CAD build for the part. Positions are in the model's coordinates, mm. A direction names the side the tool comes from. Give positions to 0.01 mm unless a question says otherwise; leave off trailing zeros. Write each loop counter-clockwise with the first axis right and the second up, starting at its lowest first coordinate (ties: lowest second). Pieces come first, ordered by that corner, then holes. Notation, with made-up numbers: (-18.75, 89) - (37.25, 89) arc R19 cw to (37.25, 107) - close; hole circle Ø5 at (34.5, 28). An arc over 180 degrees is marked (long way). Answer as a JSON object with one key per item and string values.
from build123d import *

# Parameters (mm, degrees)
F2_R     = 25.25
F3_DEPTH = 2
F5_DEPTH = 2
F6_R     = 4.99999
F7_R     = 3


# Not quite as in the source:
# - a fillet or chamfer is up to 0.001 mm smaller than in the source, because OpenCascade refuses the exact size
# - a feature names something its author has since deleted; it is built from what else it names


with BuildPart() as f1:
    # F0 (on Top) → F1 (revolve)
    with BuildSketch(Plane.XY):
        Polygon((-18, 18.5), (-18, 13.5), (0, 13.5), (11.6913429511, 20.25), (25.1913429511, 20.25), (25.1913429511, 25.25), (10.3515969889, 25.25), (-1.3397459622, 18.5), align=None)
    revolve(axis=Axis((-8.7595172226, 0, 0), (1, 0, 0)))

    # F2 (on face) → F3 (join)
    with BuildSketch(Plane.YZ.offset(25.1913429511)):
        Circle(F2_R)
    extrude(amount=F3_DEPTH)

    # F4 (on face) → F5 (cut, through all)
    with BuildSketch(Plane.YZ.offset(27.1913429511)):
        with BuildLine():
            ThreePointArc((17, 11.0028405423), (15.1695473581, 13.4144449363), (13, 15.5261875552))
            Line((13, 15.5261875552), (13, -15.5261875552))
            ThreePointArc((13, -15.5261875552), (15.1695473581, -13.4144449363), (17, -11.0028405423))
            Line((17, -11.0028405423), (17, 11.0028405423))
        make_face()
        with BuildLine():
            ThreePointArc((12, 16.3114223782), (10.0654136275, 17.5712819255), (8, 18.6027551723))
            Line((8, 18.6027551723), (8, -18.6027551723))
            ThreePointArc((8, -18.6027551723), (10.0654136275, -17.5712819255), (12, -16.3114223782))
            Line((12, -16.3114223782), (12, 16.3114223782))
        make_face()
        with BuildLine():
            ThreePointArc((7, 19.0016446657), (5.0261919098, 19.6163170571), (3, 20.0265448842))
            Line((3, 20.0265448842), (3, -20.0265448842))
            ThreePointArc((3, -20.0265448842), (5.0261919098, -19.6163170571), (7, -19.0016446657))
            Line((7, -19.0016446657), (7, 19.0016446657))
        make_face()
        with BuildLine():
            ThreePointArc((2, 20.1509925314), (0, 20.25), (-2, 20.1509925314))
            Line((-2, 20.1509925314), (-2, -20.1509925314))
            ThreePointArc((-2, -20.1509925314), (0, -20.25), (2, -20.1509925314))
            Line((2, -20.1509925314), (2, 20.1509925314))
        make_face()
        with BuildLine():
            Line((-3, -20.0265448842), (-3, 20.0265448842))
            ThreePointArc((-3, 20.0265448842), (-5.0261919098, 19.6163170571), (-7, 19.0016446657))
            Line((-7, 19.0016446657), (-7, -19.0016446657))
            ThreePointArc((-7, -19.0016446657), (-5.0261919098, -19.6163170571), (-3, -20.0265448842))
        make_face()
        with BuildLine():
            Line((-8, -18.6027551723), (-8, 18.6027551723))
            ThreePointArc((-8, 18.6027551723), (-10.0654136275, 17.5712819255), (-12, 16.3114223782))
            Line((-12, 16.3114223782), (-12, -16.3114223782))
            ThreePointArc((-12, -16.3114223782), (-10.0654136275, -17.5712819255), (-8, -18.6027551723))
        make_face()
        with BuildLine():
            Line((-13, -15.5261875552), (-13, 15.5261875552))
            ThreePointArc((-13, 15.5261875552), (-15.1695473581, 13.4144449363), (-17, 11.0028405423))
            Line((-17, 11.0028405423), (-17, -11.0028405423))
            ThreePointArc((-17, -11.0028405423), (-15.1695473581, -13.4144449363), (-13, -15.5261875552))
        make_face()
        with BuildLine():
            Line((-18, -9.2769876576), (-18, 9.2769876576))
            ThreePointArc((-18, 9.2769876576), (-20.25, 0), (-18, -9.2769876576))
        make_face()
        with BuildLine():
            ThreePointArc((20.25, 0), (19.6794626451, 4.772970773), (18, 9.2769876576))
            Line((18, 9.2769876576), (18, -9.2769876576))
            ThreePointArc((18, -9.2769876576), (19.6794626451, -4.772970773), (20.25, 0))
        make_face()
    extrude(amount=-F5_DEPTH, mode=Mode.SUBTRACT)

    # F6 (radius 5 in the source; OpenCascade refuses exactly that, so slightly less here)
    f6_edges = [f1.edges().sort_by_distance(p)[0] for p in [
        (-18, -18.5, 0),
        (-1.339746, -18.5, 0),
        (10.351597, -25.25, 0),
    ]]
    fillet(f6_edges, radius=F6_R)

    # F7
    f7_edges = [f1.edges().sort_by_distance(p)[0] for p in [
        (11.691343, -20.25, 0),
        (0, -13.5, 0),
    ]]
    fillet(f7_edges, radius=F7_R)


solid = f1.part
Item 1: Cut at A-A (x = 13.5). Give the cut face in (y, z), and give its area (3 significant figures).
Entries:
{"outline": "circle Ø50.5 at (0, 0); hole circle Ø40.5 at (0, 0)", "area": "715 mm2"}
Item 2: Mould opens along Y. For faces 4 (the cylindrical face through (19.333, 13.574, 21.291)), 5 (the flat face through (26, -18, 0)), 6 (the flat face through (26, -8, 0)) say: +Y half, -Y half, draft (parallel to the pull), parting line (faces both ways), or undercut.
Entries:
{"face 4": "parting line", "face 5": "undercut", "face 6": "undercut"}
Item 3: Cut at B-B (x = 5.5). Give the cut face in (y, z), and give its area (3 significant figures).
Entries:
{"outline": "circle Ø44.9 at (0, 0); hole circle Ø33.35 at (0, 0)", "area": "710 mm2"}
Item 4: Which spindle directions (+Z, -Z, +X, -X, +Y, -Y) get a long thin tool onto all of the face, cutting with end or side? Do faces 1 (the flat face through (26, -12, 0)), 2 (the conical face through (1.34, -3.094, -13.934)), 3 (the cylindrical face through (-9.28, -2.93, -13.18)). Say none if no direction does.
Entries:
{"face 1": "+X", "face 2": "none", "face 3": "-X"}
Item 5: Probe line 1 (Y direction, x = 18.5, z = 0); line 2 (Y direction, x = -11, z = 0). List the from-to ranges inside material, lowest first. Write a range as from..to.
Entries:
{"line 1": "-25.25..-20.25, 20.25..25.25", "line 2": "-18.5..-13.5, 13.5..18.5"}
Item 6: Flat gauge pins, fed straight in: P1, Ø2, axis at x = 26.5, z = 2, coming from the +Y side; P2, Ø1, axis at x = 26.5, z = -6.5, coming from the -Y side; P3, Ø0.6, axis at x = 26.5, z = -10, coming from the -Y side. Where does each tip first touch, or does it go through?
Entries:
{"P1": "y = 25.23", "P2": "y = -24.53", "P3": "y = -23.31"}
